```python
from build123d import *

# Parameters (mm, degrees)
SKETCH1_R                          = 6.25
BODY_DEPTH                         = 1.5
SKETCH2_R                          = 0.375
HOLE_TO_TRAP_CABLE_KNOT_DEPTH      = 10
HOLE_TO_TRAP_CABLE_KNOT_DEPTH_BACK = 7.25
THUMB_GRIP_DEPTH                   = 1.5
SKETCH13_R                         = 1.65
HOLE_FOR_SCREW_DEPTH               = 4


with BuildPart() as part:
    # Sketch1 → body (new body)
    with BuildSketch(Plane.XY):
        Circle(SKETCH1_R)
    extrude(amount=BODY_DEPTH)

    # Sketch2 → Hole to trap cable knot (cut, two sides)
    with BuildSketch(Plane(origin=(0, 0, 0), x_dir=(0, 0, -1), z_dir=(1, 0, 0))) as hole_to_trap_cable_knot_sk:
        with Locations((-0.75, 5.25)):
            Circle(SKETCH2_R)
        with Locations((-0.75, -4.75)):
            Circle(SKETCH2_R)
    extrude(amount=HOLE_TO_TRAP_CABLE_KNOT_DEPTH, mode=Mode.SUBTRACT)
    extrude(hole_to_trap_cable_knot_sk.sketch, amount=-HOLE_TO_TRAP_CABLE_KNOT_DEPTH_BACK, mode=Mode.SUBTRACT)

    # track for cable: sweep along a path in Sketch6
    with BuildLine(Plane.XY.offset(1.875)) as track_for_cable_path:
        ThreePointArc((-3.125, 5.412658774), (-0.078980905, -6.249500941), (3.260789939, 5.331955455))
    # Sketch10 → track for cable (sweep, cut)
    with BuildSketch(Plane(origin=(-5.412658774, 9.375, 0), x_dir=(-0.5, 0.866025404, 0), z_dir=(-0.866025404, -0.5, 0))):
        with BuildLine():
            Line((-4.583101682, -1.125), (-3.872701536, -1.125))
            Line((-3.872701536, -1.125), (-3.872701536, -0.374795087))
            Line((-3.872701536, -0.374795087), (-4.583101682, -0.374795087))
            ThreePointArc((-4.583101682, -0.374795087), (-4.958204138, -0.749897543), (-4.583101682, -1.125))
        make_face()
    sweep(path=track_for_cable_path.line, mode=Mode.SUBTRACT)

    # Sketch14 → thumb grip (add)
    with BuildSketch(Plane(origin=(0, 0, 0), x_dir=(-1, 0, 0), z_dir=(0, 0, -1))):
        with BuildLine():
            Line((5.729357486, 7.4822541), (2.469632038, 5.96221916))
            Line((2.469632038, 5.96221916), (1.239485083, 9.342020143))
            ThreePointArc((1.239485083, 9.342020143), (0.873368898, 9.819152044), (0.299792462, 10))
            Line((0.299792462, 10), (-0.299792462, 10))
            ThreePointArc((-0.299792462, 10), (-0.873368898, 9.819152044), (-1.239485083, 9.342020143))
            Line((-1.239485083, 9.342020143), (-2.469632038, 5.96221916))
            Line((-2.469632038, 5.96221916), (-5.729357486, 7.4822541))
            ThreePointArc((-5.729357486, 7.4822541), (-6.325623926, 7.560754066), (-6.859082529, 7.283053095))
            Line((-6.859082529, 7.283053095), (-7.283053095, 6.859082529))
            ThreePointArc((-7.283053095, 6.859082529), (-7.560754066, 6.325623926), (-7.4822541, 5.729357486))
            Line((-7.4822541, 5.729357486), (-5.96221916, 2.469632038))
            Line((-5.96221916, 2.469632038), (5.96221916, -2.469632038))
            Line((5.96221916, -2.469632038), (9.342020143, -1.239485083))
            ThreePointArc((9.342020143, -1.239485083), (9.819152044, -0.873368898), (10, -0.299792462))
            Line((10, -0.299792462), (10, 0.299792462))
            ThreePointArc((10, 0.299792462), (9.819152044, 0.873368898), (9.342020143, 1.239485083))
            Line((9.342020143, 1.239485083), (5.96221916, 2.469632038))
            Line((5.96221916, 2.469632038), (7.4822541, 5.729357486))
            ThreePointArc((7.4822541, 5.729357486), (7.560754066, 6.325623926), (7.283053095, 6.859082529))
            Line((7.283053095, 6.859082529), (6.859082529, 7.283053095))
            ThreePointArc((6.859082529, 7.283053095), (6.325623926, 7.560754066), (5.729357486, 7.4822541))
        make_face()
    extrude(amount=THUMB_GRIP_DEPTH)

    # Sketch13 → hole for screw (cut, through all)
    with BuildSketch(Plane.XY.offset(1.5)):
        Circle(SKETCH13_R)
    extrude(amount=-HOLE_FOR_SCREW_DEPTH, mode=Mode.SUBTRACT)

    # Sketch20 → trap for ball (revolve, cut)
    with BuildSketch(Plane(origin=(3.1, 0, 0), x_dir=(0, 0, -1), z_dir=(1, 0, 0))):
        with BuildLine():
            Line((-0.75, 7), (-0.75, 3.5))
            ThreePointArc((-0.75, 3.5), (1, 5.25), (-0.75, 7))
        make_face()
    revolve(axis=Axis((3.1, 7.793428849, 0.75), (0, -1, 0)), mode=Mode.SUBTRACT)


solid = part.part
```
Geometry check sheet. Reference: the model listing, model coordinates, mm. A direction names the side the tool comes from. Coordinates: 2 decimals unless noted, no trailing zeros. Write each loop counter-clockwise with the first axis right and the second up, starting at its lowest first coordinate (ties: lowest second). Pieces come first, ordered by that corner, then holes. Notation, with made-up numbers: M 6,-12.5 L 37,-12.5 A17 ccw 37,-8.5 Z; hole C -38.5,12.5 d10. An arc over 180 degrees is marked long. Use one line per item in the form item = value. Start each with the question number.
1) Release check for a two-part mould opening along X. For faces 1 (the flat face through (-4.12, 6.73, -0.74)), 2 (the flat face through (1.3, -1.3, 1.5)), 3 (the flat face through (-1.863, 7.628, -0.74)), 4 (the flat face through (-3.712, -1.538, -0.74)) record: pulls with the +X half, pulls with the -X half, needs draft (parallel to the pull), parting line crosses it, or undercut.
2) Set-up check for faces 5 (the flat face through (1, -3, 0)), 6 (the flat face through (6, 6, 0)), 7 (the flat face through (-7.628, -1.863, -0.74)), 8 (the cylindrical face through (-0.02, 6.25, 0.74)), 9 (the flat face through (-6.712, 4.077, -0.74)): record each of +Z, -Z, +X, -X, +Y, -Y from which the full face is reachable in a straight line by a thin tool's end or side.
3) Section check B-B on x = 0. State how many separate pieces and enclosed holes the cut face has, and give its area (3 significant figures).
4) Section check A-A on z = 0.75. Enter the section's corners in (x, y) (3 decimals), and give its area (3 significant figures).
5) Go/stop test with flat-tipped pins: pin 1 Ø1.1 at (x, y) = (5.5, 4.5) entering from +Z; pin 2 Ø1 at (y, z) = (-4.5, 0) entering from +X; pin 3 Ø7 at (x, y) = (0, -4) entering from -Z. Record where each tip stops, or that it passes through.
6) Thickness scan on probe 1 along X at (y, z) = (0, 0.25); probe 2 along Z at (x, y) = (0, -4.75) (3 decimals); probe 3 along Z at (x, y) = (0.2, 5.25) (3 decimals). Record the ranges inside material, lowest first. Write a range as from..to.
Responses:
q1.face_1 = undercut
q1.face_2 = needs draft
q1.face_3 = undercut
q1.face_4 = pulls with the +X half
q2.face_5 = -Z, +X, -Y
q2.face_6 = +Z, +X, +Y
q2.face_7 = +Z, -Z, -X, -Y
q2.face_8 = +Z
q2.face_9 = +Z, -Z, -X
q3.separate_pieces = 2
q3.enclosed_holes = 2
q3.area = 25.2 mm2
q4.outline = M -3.909,-4.375 L 3.909,-4.375 A5.867 ccw 4.308,3.983 A1.75 cw 1.391,4.875 L -3.265,4.875 A5.867 ccw Z; M -2.856,-5.125 A5.867 ccw 2.856,-5.125 Z; M -2.724,5.625 L 1.391,5.625 A1.75 cw 1.546,6.056 A6.25 ccw Z; hole C 0,0 d3.3
q4.area = 89.2 mm2
q5.pin_1 = 0
q5.pin_2 = 4.8
q5.pin_3 = 0
q6.probe_1 = -6.25..-1.65, 1.65..6.25
q6.probe_2 = 0..0.375, 1.125..1.5
q6.probe_3 = -1.5..0.375, 1.125..1.5
